Verification items for the finished model (mm, model axes). A direction names the side the tool comes from. Coordinates: 2 decimals unless noted, no trailing zeros. Write each loop counter-clockwise with the first axis right and the second up, starting at its lowest first coordinate (ties: lowest second). Pieces come first, ordered by that corner, then holes. Notation, with made-up numbers: (-18.75, 23) -> (-6.75, 23) arc R10 cw to (-6.75, 36) -> close; hole circle Ø11 at (68, 38.25). An arc over 180 degrees is marked (long way). Use CSV: the item, a comma, the result in double quotes.
```python
from build123d import *

# Parameters (mm, degrees)
F0_W     = 29
F0_H     = 4.9
F0_H_2   = 5.5
F0_R     = 1
F0_H_3   = 5
F1_DEPTH = 2
F2_DEPTH = 25
F3_R     = 1
F4_DEPTH = 25
F3_R_2   = 3.5
F5_DEPTH = 13
F6_R     = 2


with BuildPart() as f1:
    # F0 (on Top) → F1 (new body)
    with BuildSketch(Plane.XY):
        with Locations((0, -7.95)):
            Rectangle(F0_W, F0_H)
        with Locations((0, -2.75)):
            Rectangle(F0_W, F0_H_2)
        with Locations((0, -3)):
            Circle(F0_R, mode=Mode.SUBTRACT)
        with Locations((0, 2.5)):
            Rectangle(F0_W, F0_H_3)
    extrude(amount=F1_DEPTH)

    # F0 (on Top) → F2 (join)
    with BuildSketch(Plane.XY):
        with Locations((0, -7.95)):
            Rectangle(F0_W, F0_H)
        with Locations((0, 2.5)):
            Rectangle(F0_W, F0_H_3)
    extrude(amount=F2_DEPTH)

    # F3 (on face) → F4 (cut)
    with BuildSketch(Plane.XZ.offset(10.4)):
        with Locations((6, 9.462781)):
            Circle(F3_R)
        with Locations((-6, 9.462781)):
            Circle(F3_R)
    extrude(amount=-F4_DEPTH, mode=Mode.SUBTRACT)

    # F3 (on face) → F5 (cut)
    with BuildSketch(Plane.XZ.offset(10.4)):
        with Locations((-6, 9.462781)):
            Circle(F3_R_2)
        with Locations((-6, 9.462781)):
            Circle(F3_R, mode=Mode.SUBTRACT)
        with Locations((6, 9.462781)):
            Circle(F3_R_2)
        with Locations((6, 9.462781)):
            Circle(F3_R, mode=Mode.SUBTRACT)
    extrude(amount=-F5_DEPTH, mode=Mode.SUBTRACT)

    # F6
    f6_edges = [f1.edges().sort_by_distance(p)[0] for p in [
        (0, -10.4, 0),
    ]]
    fillet(f6_edges, radius=F6_R)


solid = f1.part
```
1) Cross-section at B-B (x = -6). Record the boundary of the cut face in (y, z), plus the area to 3 significant figures.
Return value:
outline,"(-10.4, 2) arc R2 ccw to (-8.4, 0) -> (5, 0) -> (5, 8.46) -> (2.6, 8.46) -> (2.6, 5.96) -> (0, 5.96) -> (0, 2) -> (-5.5, 2) -> (-5.5, 5.96) -> (-10.4, 5.96) -> close; (-10.4, 12.96) -> (-5.5, 12.96) -> (-5.5, 25) -> (-10.4, 25) -> close; (0, 12.96) -> (2.6, 12.96) -> (2.6, 10.46) -> (5, 10.46) -> (5, 25) -> (0, 25) -> close"
area,"200 mm2"
2) Cross-section at A-A (y = -3). Record the boundary of the cut face in (x, z).
Return value:
outline,"(-14.5, 0) -> (-1, 0) -> (-1, 2) -> (-14.5, 2) -> close; (1, 0) -> (14.5, 0) -> (14.5, 2) -> (1, 2) -> close"
3) Cross-section at D-D (x = 5.5). Record the boundary of the cut face in (y, z), plus the area to 3 significant figures.
Return value:
outline,"(-10.4, 2) arc R2 ccw to (-8.4, 0) -> (5, 0) -> (5, 8.6) -> (2.6, 8.6) -> (2.6, 6) -> (0, 6) -> (0, 2) -> (-5.5, 2) -> (-5.5, 6) -> (-10.4, 6) -> close; (-10.4, 12.93) -> (-5.5, 12.93) -> (-5.5, 25) -> (-10.4, 25) -> close; (0, 12.93) -> (2.6, 12.93) -> (2.6, 10.33) -> (5, 10.33) -> (5, 25) -> (0, 25) -> close"
area,"202 mm2"
4) Mould release check, pull along Z, two halves, no side actions. Record for faces 4 (the cylindrical face through (-4.1, -8, 12.4)), 5 (the flat face through (5.2, 2.6, 10.3)), 6 (the flat face through (0, -10.4, 13)), 7 (the flat face through (0, -8, 25)): released by +Z, released by -Z, zero draft, split by the parting line, or undercut.
Return value:
face 4,"undercut"
face 5,"undercut"
face 6,"zero draft"
face 7,"released by +Z"
5) Cross-section at C-C (z = 15). Record the boundary of the cut face in (x, y).
Return value:
outline,"(-14.5, -10.4) -> (14.5, -10.4) -> (14.5, -5.5) -> (-14.5, -5.5) -> close; (-14.5, 0) -> (14.5, 0) -> (14.5, 5) -> (-14.5, 5) -> close"
6) Scan lines: L1, parallel to Y at x = -5.75, z = 21.25; L2, parallel to Z at x = -6, y = -7.8; L3, parallel to X at y = 1, z = 11.25. Record each from-to range of solid material in increasing order.
Return value:
L1,"-10.4 to -5.5, 0 to 5"
L2,"0 to 5.96, 12.96 to 25"
L3,"-14.5 to -9.01, -2.99 to 2.99, 9.01 to 14.5"
7) Set-up check for faces 1 (the flat face through (-6.8, 2.6, 10.3)), 2 (the flat face through (0, 5, 12)), 3 (the flat face through (0, -5.5, 13)): record each of +Z, -Z, +X, -X, +Y, -Y from which the full face is reachable in a straight line by a thin tool's end or side.
Return value:
face 1,"-Y"
face 2,"+Z, -Z, +X, -X, +Y"
face 3,"+Z, +X, -X"
8) Gauge pin test, flat ends, axial feed: pin 1 (1.6 mm diameter, centred on x = -1, y = -2.5, fed in from +Z); pin 2 (5.5 mm diameter, centred on x = 6, z = 9.46, fed in from -Y). Record the tip position at first contact, or that the pin passes through.
Return value:
pin 1,"z = 2"
pin 2,"y = 2.6"
